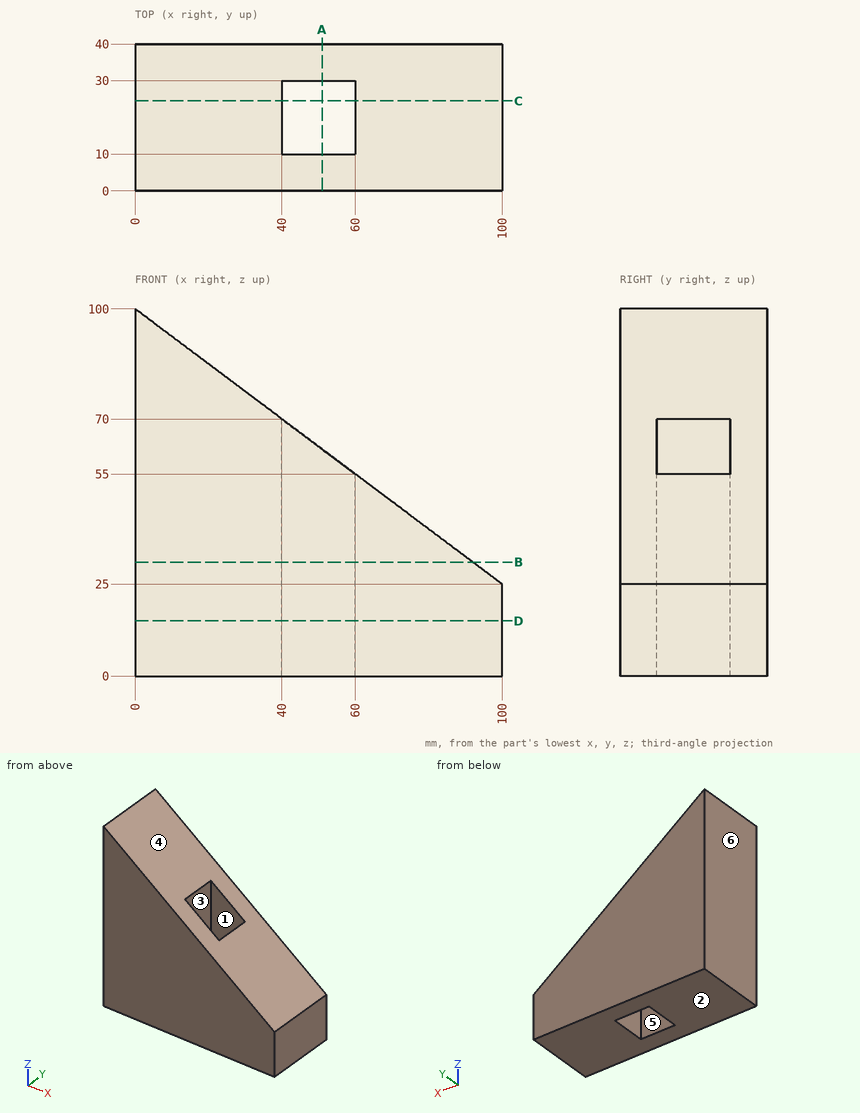
Job drawing, mm, ordinate dimensions from the low corner. One solid piece. A direction names the side the tool comes from. Round coordinates to 2 decimals unless told otherwise and drop trailing zeros. Write each loop counter-clockwise with the first axis right and the second up, starting at its lowest first coordinate (ties: lowest second). Pieces come first, ordered by that corner, then holes.
1) Drill centre lines: probe 1 along X at (y, z) = (22, 13); probe 2 along Y at (x, z) = (45.5, 39); probe 3 along X at (y, z) = (20, 44). Where is each one in solid material? Low to high.
2) 3-axis set-ups, long thin cutter, end or side, ignore diameter. For the marked faces 5 and 6: which of +Z, -Z, +X, -X, +Y, -Y reach the whole face in a straight line?
3) Band-saw the part on D-D, the plane z = 15. List the corners of the cut face in (x, y).
4) Mould opens along X. For the marked faces 1, 2, 3 and 4 say: +X half, -X half, draft (parallel to the pull), parting line (faces both ways), or undercut.
5) Band-saw the part on B-B, the plane z = 31. List the corners of the cut face in (x, y).
6) Band-saw the part on C-C, the plane y = 24.5. List the corners of the cut face in (x, z).
7) Pin check, flat tips, straight feed: pin 1 (6 mm diameter, centred on y = 18.5, z = 35.5, fed in from -X); pin 2 (2 mm diameter, centred on y = 31, z = 47.5, fed in from +X); pin 3 (5 mm diameter, centred on y = 22.5, z = 46.5, fed in from +X); pin 4 (6 mm diameter, centred on y = 23, z = 37, fed in from +X). Stop position of each tip, or through.
8) Band-saw the part on A-A, the plane x = 51. List the corners of the cut face in (y, z), and give its area (4 significant figures).
Ans:
1. probe 1: x = 0 to 40, 60 to 100
1. probe 2: y = 0 to 10, 30 to 40
1. probe 3: x = 0 to 40, 60 to 74.67
2. face 5: +Z, -Z
2. face 6: +Z, -Z, -X, +Y, -Y
3. outline: (0, 0) - (100, 0) - (100, 40) - (0, 40) - close; hole (40, 10) - (60, 10) - (60, 30) - (40, 30) - close
4. face 1: undercut
4. face 2: draft
4. face 3: undercut
4. face 4: +X half
5. outline: (0, 0) - (92, 0) - (92, 40) - (0, 40) - close; hole (40, 10) - (60, 10) - (60, 30) - (40, 30) - close
6. outline: (0, 0) - (40, 0) - (40, 70) - (0, 100) - close; (60, 0) - (100, 0) - (100, 25) - (60, 55) - close
7. pin 1: stops at x = 0
7. pin 2: stops at x = 71.33
7. pin 3: stops at x = 74.67
7. pin 4: stops at x = 88
8. outline: (0, 0) - (10, 0) - (10, 61.75) - (0, 61.75) - close; (30, 0) - (40, 0) - (40, 61.75) - (30, 61.75) - close
8. area: 1,235 mm2
